Input: part model. Units: mm. Frame: model coordinates. Round coordinates to 2 decimals unless told otherwise and drop trailing zeros. Loops run counter-clockwise (first coordinate to the right, second up) from the corner with the lowest first, then second, coordinate; pieces in that order, holes last.
1) First-contact query: pin 1 (0.6 mm diameter, centred on y = 11, z = 1, fed in from +X); pin 2 (0.6 mm diameter, centred on x = -21, z = 1, fed in from +Y); pin 3 (1 mm diameter, centred on x = -23, z = 1.5, fed in from -Y). Flat tips, straight axial feed; report the tip coordinate or a pass-through.
2) Section C-C, the plane x = -6. Return loops of the section in (y, z), and give its area (3 significant figures).
3) Ray query, line 1 along Y through (x, z) = (-49, 0.1); line 2 along X through (y, z) = (-17, 1.1); line 3 along Y through (x, z) = (-13.5, 1.8). Return the intervals inside material, ascending.
4) Section A-A, the plane z = 0.5. Return loops of the section in (x, y), and give its area (3 significant figures).
5) Section B-B, the plane y = -19. Return loops of the section in (x, z).
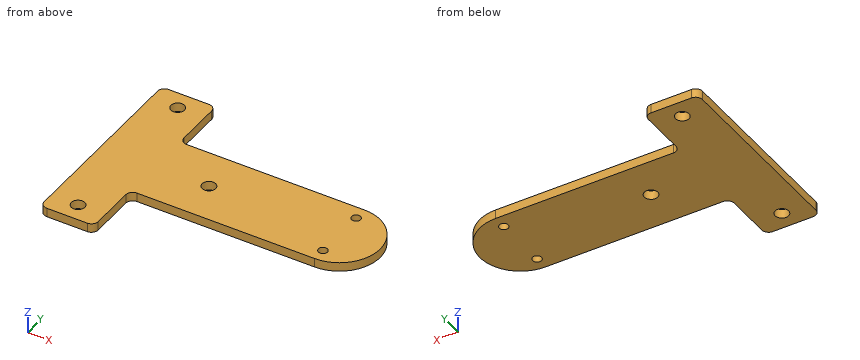
from build123d import *

# Parameters (mm, degrees)
SKETCH_1_R      = 1.5
SKETCH_1_R_2    = 1
EXTRUDE_1_DEPTH = 2
FILLET_1_R      = 1.5


with BuildPart() as part:
    # 草图1 → 凸台-拉伸1 (new body)
    with BuildSketch(Plane.XY):
        with BuildLine():
            Line((-1.723571429, -13.369911995), (-42.723571429, -13.369911995))
            Line((-42.723571429, -13.369911995), (-42.723571429, -26.369911995))
            Line((-42.723571429, -26.369911995), (-54.723571429, -26.369911995))
            Line((-54.723571429, -26.369911995), (-54.723571429, 17.630088005))
            Line((-54.723571429, 17.630088005), (-42.723571429, 17.630088005))
            Line((-42.723571429, 17.630088005), (-42.723571429, 4.630088005))
            Line((-42.723571429, 4.630088005), (-1.723571429, 4.630088005))
            ThreePointArc((-1.723571429, 4.630088005), (7.276428571, -4.369911995), (-1.723571429, -13.369911995))
        make_face()
        with Locations((-30.723571429, -4.369911995)):
            Circle(SKETCH_1_R, mode=Mode.SUBTRACT)
        with Locations((-48.723571429, 13.630088005)):
            Circle(SKETCH_1_R, mode=Mode.SUBTRACT)
        with Locations((-48.723571429, -22.369911995)):
            Circle(SKETCH_1_R, mode=Mode.SUBTRACT)
        with Locations((-1.723571429, 1.630088005)):
            Circle(SKETCH_1_R_2, mode=Mode.SUBTRACT)
        with Locations((-1.723571429, -10.369911995)):
            Circle(SKETCH_1_R_2, mode=Mode.SUBTRACT)
    extrude(amount=EXTRUDE_1_DEPTH)

    # 圆角1
    fillet_1_edges = [part.edges().sort_by_distance(p)[0] for p in [
        (-42.723571429, -13.369911995, 1),
        (-42.723571429, -26.369911995, 1),
        (-54.723571429, -26.369911995, 1),
        (-54.723571429, 17.630088005, 1),
        (-42.723571429, 17.630088005, 1),
        (-42.723571429, 4.630088005, 1),
    ]]
    fillet(fillet_1_edges, radius=FILLET_1_R)


solid = part.part
Final values:
1. pin 1: stops at x = -42.72
1. pin 2: stops at y = 4.63
1. pin 3: stops at y = -13.37
2. outline: (-13.37, 0) - (4.63, 0) - (4.63, 2) - (-13.37, 2) - close
2. area: 36.0 mm2
3. line 1: y = -26.37 to -23.84, -20.9 to 12.16, 15.1 to 17.63
3. line 2: x = -54.72 to -42.72
3. line 3: y = -13.37 to 4.63
4. outline: (-54.72, -24.87) arc R1.5 ccw to (-53.22, -26.37) - (-44.22, -26.37) arc R1.5 ccw to (-42.72, -24.87) - (-42.72, -14.87) arc R1.5 cw to (-41.22, -13.37) - (-1.72, -13.37) arc R9 ccw to (-1.72, 4.63) - (-41.22, 4.63) arc R1.5 cw to (-42.72, 6.13) - (-42.72, 16.13) arc R1.5 ccw to (-44.22, 17.63) - (-53.22, 17.63) arc R1.5 ccw to (-54.72, 16.13) - close; hole circle Ø3 at (-48.72, -22.37); hole circle Ø3 at (-48.72, 13.63); hole circle Ø3 at (-30.72, -4.37); hole circle Ø2 at (-1.72, -10.37); hole circle Ø2 at (-1.72, 1.63)
4. area: 1,360 mm2
5. outline: (-54.72, 0) - (-42.72, 0) - (-42.72, 2) - (-54.72, 2) - close
